The drawing under review shows one solid part. Ordinate dimensions are in mm from its lowest x, y, z. A direction names the side the tool comes from. Give positions to 0.01 mm unless a question says otherwise; leave off trailing zeros. Loops run counter-clockwise (first coordinate to the right, second up) from the corner with the lowest first, then second, coordinate; pieces in that order, holes last. Notation, with made-up numbers: (26, -9.75) - (69, -9.75) arc R33 cw to (69, 21.25) - close; hole circle Ø3 at (9.5, 43). An arc over 180 degrees is marked (long way). Return JSON: item names as keys, results as strings. Group by question number.
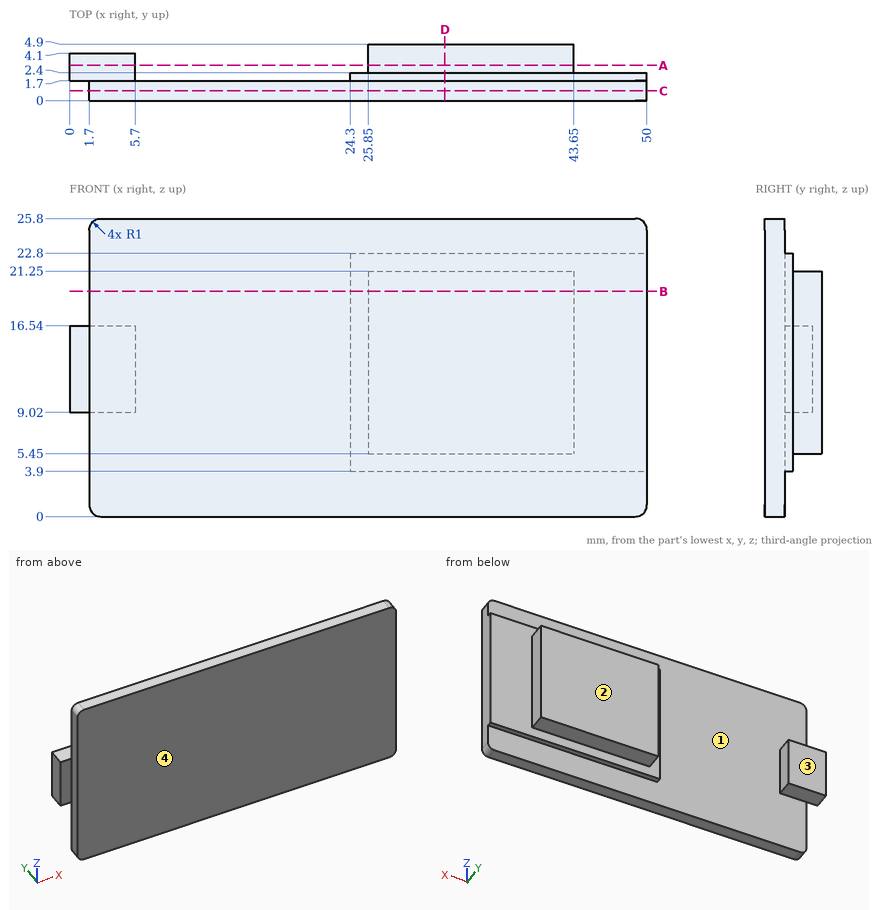
1) We need section D-D, the plane x = 32.5. Write out the cut boundary in (y, z), plus the area to 3 significant figures.
2) Tool access review of the marked faces 3 and 4: name each direction out of +Z, -Z, +X, -X, +Y, -Y from which nothing blocks a thin tool from reaching the whole face with its end or side.
3) We need section A-A, the plane y = 3.05. Write out the cut boundary in (x, z).
4) We need section B-B, the plane z = 19.5. Write out the cut boundary in (x, y), plus the area to 3 significant figures.
5) We need section C-C, the plane y = 0.85. Write out the cut boundary in (x, z).
6) To check wall thickness, follow line 1 (X direction, y = 2.45, z = 14.5); line 2 (Y direction, x = 23.5, z = 3.5); line 3 (Z direction, x = 43.5, y = 3.95). State the ranges of each line that lie inside material, in increasing order.
7) Draft analysis for pull direction X (two halves, no side actions). For the marked faces 1 and 2, state which applies: +X half, -X half, draft (parallel to the pull), parting line (faces both ways), or undercut.
8) For pin 1 Ø1.7 at (x, z) = (2.5, 14) entering from +Y; pin 2 Ø0.8 at (y, z) = (1, 12) entering from -X; pin 3 Ø0.7 at (x, y) = (2.5, 3.5) entering from +Z, all flat-tipped, find the tip position at first contact; note any pin that passes through.
Findings:
{
 "1": {"outline": "(0, 0) - (1.7, 0) - (1.7, 3.9) - (2.4, 3.9) - (2.4, 5.45) - (4.9, 5.45) - (4.9, 21.25) - (2.4, 21.25) - (2.4, 22.8) - (1.7, 22.8) - (1.7, 25.8) - (0, 25.8) - close", "area": "96.6 mm^2"},
 "2": {"face 3": "+Z, -Z, -X, +Y", "face 4": "+Z, -Z, +X, -X, -Y"},
 "3": {"outline": "(0, 9.02) - (5.7, 9.02) - (5.7, 16.54) - (0, 16.54) - close; (25.85, 5.45) - (43.65, 5.45) - (43.65, 21.25) - (25.85, 21.25) - close"},
 "4": {"outline": "(1.7, 0) - (50, 0) - (50, 2.4) - (43.65, 2.4) - (43.65, 4.9) - (25.85, 4.9) - (25.85, 2.4) - (24.3, 2.4) - (24.3, 1.7) - (1.7, 1.7) - close", "area": "145 mm^2"},
 "5": {"outline": "(1.7, 1) arc R1 ccw to (2.7, 0) - (49, 0) arc R1 ccw to (50, 1) - (50, 24.8) arc R1 ccw to (49, 25.8) - (2.7, 25.8) arc R1 ccw to (1.7, 24.8) - close"},
 "6": {"line 1": "x = 0 to 5.7, 25.85 to 43.65", "line 2": "y = 0 to 1.7", "line 3": "z = 5.45 to 21.25"},
 "7": {"face 1": "undercut", "face 2": "draft"},
 "8": {"pin 1": "stops at y = 4.1", "pin 2": "stops at x = 1.7", "pin 3": "stops at z = 16.54"}
}
